Geometry: see drawing. Coordinates: mm, zero at the bounding-box minimum. Round coordinates to 2 decimals unless told otherwise and drop trailing zeros. Order: outer loops, then holes, each group sorted by start corner. A loop starts at its lowest first (then second) coordinate and runs counter-clockwise, first axis right, second up. Notation, with made-up numbers: (18, 89) -> (61, 89) arc R18 cw to (61, 109) -> close; hole circle Ø1 at (-26, 36.5). An arc over 180 degrees is marked (long way). Answer as CSV lines item,"result". Start each with the question number.
(1) Section query B-B (y = 31). Output: boundary loops of the cut face in (x, z), plus the area to 3 significant figures.
(2) Line query: line 1 along Z through (x, y) = (30.5, 5); line 2 along Y through (x, z) = (26.5, 36); line 3 along Y through (x, z) = (27.5, 36). Output: solid intervals per line, ascending. Write a range as from..to.
(3) Contact query for flat-ended pins moving along their axis: P1, Ø6, axis at x = 6, y = 12, coming from the +Z side; P2, Ø1, axis at x = 32.5, z = 31, coming from the -Y side; P3, Ø12, axis at y = 10, z = 17.5, coming from the -X side. Output: stop coordinate, or through.
(4) Section query D-D (y = 19). Output: boundary loops of the cut face in (x, z), plus the area to 3 significant figures.
(5) Section query C-C (z = 21). Output: boundary loops of the cut face in (x, y), plus the area to 3 significant figures.
(6) Section query A-A (x = 19). Output: boundary loops of the cut face in (y, z).
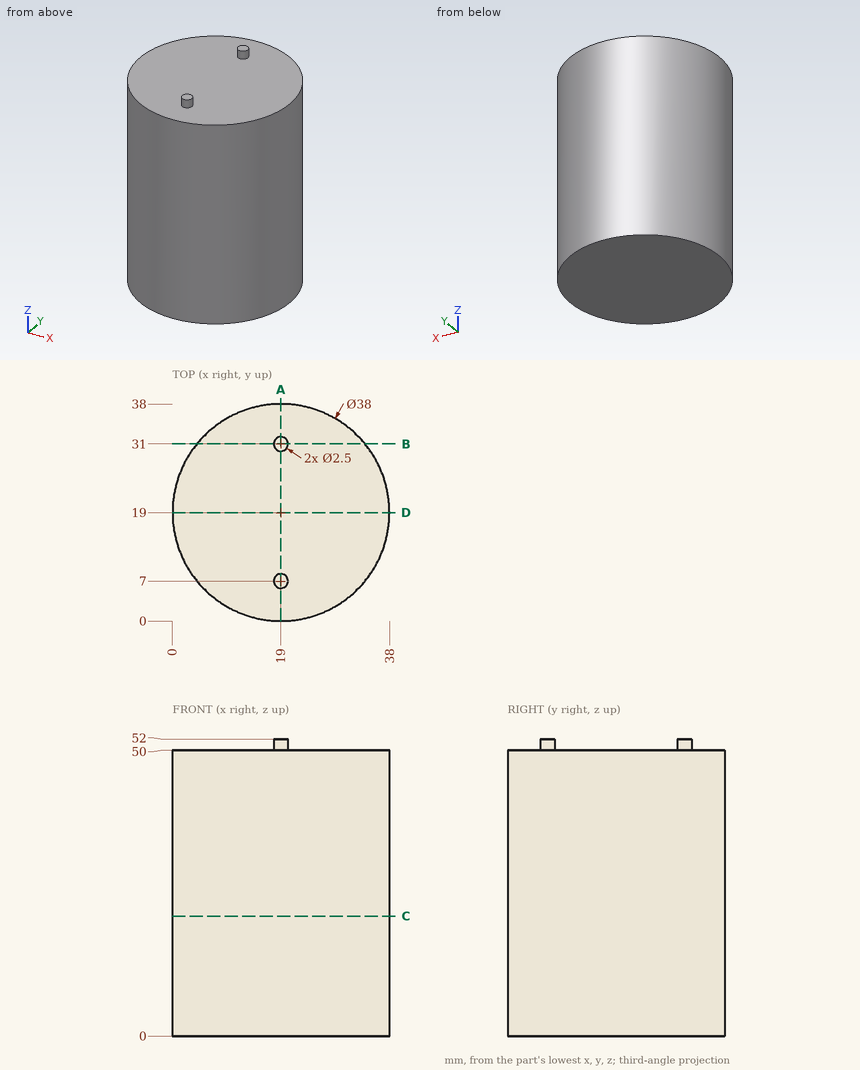
Answer block:
1,outline,"(4.27, 0) -> (33.73, 0) -> (33.73, 50) -> (20.25, 50) -> (20.25, 52) -> (17.75, 52) -> (17.75, 50) -> (4.27, 50) -> close"
1,area,"1,480 mm2"
2,line 1,"0..50"
2,line 2,"1.54..36.46"
2,line 3,"2.01..35.99"
3,P1,"z = 50"
3,P2,"y = 5.14"
3,P3,"x = 0.24"
4,outline,"(0, 0) -> (38, 0) -> (38, 50) -> (0, 50) -> close"
4,area,"1,900 mm2"
5,outline,"circle Ø38 at (19, 19)"
5,area,"1,130 mm2"
6,outline,"(0, 0) -> (38, 0) -> (38, 50) -> (32.25, 50) -> (32.25, 52) -> (29.75, 52) -> (29.75, 50) -> (8.25, 50) -> (8.25, 52) -> (5.75, 52) -> (5.75, 50) -> (0, 50) -> close"
